Check sheet for the modelled part. Datum: model origin and axes. Units: mm. Face numbers are marked on the shaded views. Round coordinates to 2 decimals unless told otherwise and drop trailing zeros. Order: outer loops, then holes, each group sorted by start corner. A loop starts at its lowest first (then second) coordinate and runs counter-clockwise, first axis right, second up. Notation, with made-up numbers: (-25, 1.25) -> (-9, 1.25) arc R22 cw to (-9, 32.25) -> close; hole circle Ø2 at (68, 65.5). An arc over 180 degrees is marked (long way). Use CSV: the item, a comma, the result in double quotes.
```python
from build123d import *

# Parameters (mm, degrees)
SKETCH_1_R          = 12.5
EXTRUDE_1_DEPTH     = 145
SKETCH_2_W          = 70.200911856
SKETCH_2_H          = 10
CUT_EXTRUDE_2_DEPTH = 30
SKETCH_4_R          = 2.5
CUT_EXTRUDE_1_DEPTH = 35
SKETCH_5_W          = 33.79642712
SKETCH_5_H          = 6.499312907
CUT_EXTRUDE_4_DEPTH = 30


with BuildPart() as part:
    # Эскиз1 → Вытянуть1 (new body)
    with BuildSketch(Plane.XY):
        Circle(SKETCH_1_R)
    extrude(amount=EXTRUDE_1_DEPTH)

    # Эскиз2 → Вытянуть2 (cut)
    with BuildSketch(Plane(origin=(0, 0, 0), x_dir=(-1, 0, 0), z_dir=(0, 0, -1))):
        Rectangle(SKETCH_2_W, SKETCH_2_H)
    extrude(amount=-CUT_EXTRUDE_2_DEPTH, mode=Mode.SUBTRACT)

    # Эскиз4 → Вырез-Вытянуть1 (cut, symmetric)
    with BuildSketch(Plane(origin=(0, 0, 0), x_dir=(1, 0, 0), z_dir=(0, 1, 0))):
        with Locations(Location((0, -5.680597097, 0), (0, 0, 270))):
            Circle(SKETCH_4_R)
        with Locations(Location((0, -15.185844734, 0), (0, 0, 270))):
            Circle(SKETCH_4_R)
        with Locations(Location((0, -24.408758256, 0), (0, 0, 270))):
            Circle(SKETCH_4_R)
    extrude(amount=CUT_EXTRUDE_1_DEPTH, both=True, mode=Mode.SUBTRACT)

    # Эскиз5 → Вытянуть4 (cut)
    with BuildSketch(Plane(origin=(0, 0, 0), x_dir=(-1, 0, 0), z_dir=(0, 0, -1))):
        with Locations((0.724923363, -14.423475184)):
            Rectangle(SKETCH_5_W, SKETCH_5_H)
        with Locations((0.724923363, 14.423475184)):
            Rectangle(SKETCH_5_W, SKETCH_5_H)
    extrude(amount=-CUT_EXTRUDE_4_DEPTH, mode=Mode.SUBTRACT)


solid = part.part
```
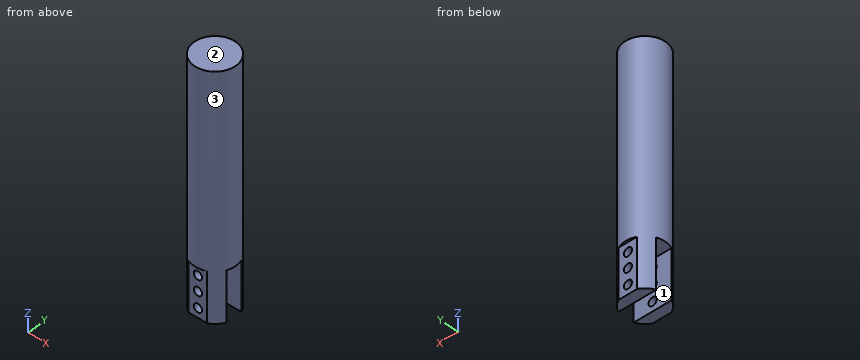
Q1. Scan lines: L1, parallel to Y at x = -2.5, z = 11.5; L2, parallel to Z at x = 3.25, y = -3.75; L3, parallel to Y at x = -8.25, z = 19. Record each from-to range of solid material in increasing order.
Result sheet:
L1,"y = -11.17 to -5, 5 to 11.17"
L2,"z = 30 to 145"
L3,"y = -9.39 to -5, 5 to 9.39"
Q2. Sectioned sample at B-B, the plane x = 7.5. Enter the section's corners in (y, z), then the cut area to 3 significant figures.
Result sheet:
outline,"(-10, 0) -> (-5, 0) -> (-5, 30) -> (5, 30) -> (5, 0) -> (10, 0) -> (10, 145) -> (-10, 145) -> close"
area,"2,600 mm^2"
Q3. Sectioned sample at C-C, the plane y = 0. Enter the section's corners in (x, z), then the cut area to 4 significant figures.
Result sheet:
outline,"(-12.5, 30) -> (12.5, 30) -> (12.5, 145) -> (-12.5, 145) -> close"
area,"2,875 mm^2"
Q4. Sectioned sample at D-D, the plane y = -8.5. Enter the section's corners in (x, z), then the cut area to 3 significant figures.
Result sheet:
outline,"(-9.17, 0) -> (9.17, 0) -> (9.17, 145) -> (-9.17, 145) -> close; hole circle Ø5 at (0, 5.68); hole circle Ø5 at (0, 15.19); hole circle Ø5 at (0, 24.41)"
area,"2,600 mm^2"
Q5. Mould release check, pull along Y, two halves, no side actions. Record for the marked faces 1, 2 and 3: pulls with the +Y half, pulls with the -Y half, needs draft (parallel to the pull), parting line crosses it, or undercut.
Result sheet:
face 1,"undercut"
face 2,"needs draft"
face 3,"parting line crosses it"
Q6. Sectioned sample at A-A, the plane z = 28.5. Enter the section's corners in (x, y), then the cut area to 3 significant figures.
Result sheet:
outline,"(-11.46, -5) arc R12.5 ccw to (-5.6, -11.17) -> (5.6, -11.17) arc R12.5 ccw to (11.46, -5) -> close; (-11.46, 5) -> (11.46, 5) arc R12.5 ccw to (5.6, 11.17) -> (-5.6, 11.17) arc R12.5 ccw to start"
area,"228 mm^2"
Q7. Go/stop test with flat-tipped pins: pin 1 (2 mm diameter, centred on y = 6, z = 49, fed in from -X); pin 2 (12 mm diameter, centred on x = 6.5, z = 40.5, fed in from -Y); pin 3 (6 mm diameter, centred on x = 0, z = 15.19, fed in from +Y). Record where each tip stops, or that it passes through.
Result sheet:
pin 1,"stops at x = -11.46"
pin 2,"stops at y = -12.49"
pin 3,"stops at y = 11.17"
